Verification items for the finished model (mm, model axes). A direction names the side the tool comes from. Coordinates: 2 decimals unless noted, no trailing zeros. Order: outer loops, then holes, each group sorted by start corner. A loop starts at its lowest first (then second) coordinate and runs counter-clockwise, first axis right, second up. Notation, with made-up numbers: M 24,78 L 56,78 A22 ccw 56,86 Z; hole C 5.5,-30 d8. An arc over 180 degrees is marked long. Return JSON: item names as keys, results as strings. Group by question number.
1. Material ranges on line 1 along Y through (x, z) = (14.75, 5.75); line 2 along X through (y, z) = (5, 5); line 3 along Y through (x, z) = (-2, 6.5), recorded low to high.
2. Mould release check, pull along X, two halves, no side actions. Record for faces 5 (the cylindrical face through (-2, 10.5, 5)), 6 (the flat face through (8, 9, 0)), 7 (the flat face through (10, 16, 4)): +X half, -X half, draft (parallel to the pull), parting line (faces both ways), or undercut.
3. Section check C-C, the plane z = 1.75. Record the cut outline in (x, y), plus the area to 3 significant figures.
4. Section check B-B, the plane y = 12. Record the cut outline in (x, z), plus the area to 3 significant figures.
5. Gauge pin test, flat ends, axial feed: pin 1 (4 mm diameter, centred on y = 3.5, z = 2.5, fed in from +X); pin 2 (2.5 mm diameter, centred on x = -1.7, z = 4.15, fed in from -Y); pin 3 (4.5 mm diameter, centred on x = -1.5, z = 3.5, fed in from +Y). Record the tip position at first contact, or that the pin passes through.
6. Section check D-D, the plane x = 4. Record the cut outline in (y, z), plus the area to 3 significant figures.
7. Section check A-A, the plane x = 11.75. Record the cut outline in (y, z).
8. Set-up check for faces 1 (the flat face through (16.1, 5, 4)), 2 (the flat face through (0, 14, 4)), 3 (the flat face through (13, 14.6, 4)), 4 (the flat face through (0, 5, 4)): record each of +Z, -Z, +X, -X, +Y, -Y from which the full face is reachable in a straight line by a thin tool's end or side.
```python
from build123d import *

# Parameters (mm, degrees)
EXTRUDE_1_DEPTH     = 8.3
SKETCH_9_R          = 1.8
EXTRUDE_6_DEPTH     = 3
CHAMFER_1_SIZE      = 0.3
EXTRUDE_7_DEPTH     = 0.5
SKETCH_11_R         = 0.9
CUT_EXTRUDE_1_DEPTH = 10


with BuildPart() as part:
    # 草图1 → 凸台-拉伸1 (new body)
    with BuildSketch(Plane.XY):
        Polygon((16.1, 10.2), (17.8, 10.2), (17.8, 10.7), (16.1, 10.7), (16.1, 14.6), (10, 14.6), (10, 17.2), (0, 17.2), (0, 10.7), (-1.7, 10.7), (-1.7, 10.2), (0, 10.2), (0, 0), (16.1, 0), align=None)
    extrude(amount=EXTRUDE_1_DEPTH)

    # 草图9 → 凸台-拉伸6 (add)
    with BuildSketch(Plane(origin=(0, 17.2, 0), x_dir=(1, 0, 0), z_dir=(0, 1, 0))):
        with Locations(Location((4, -4, 0), (0, 0, 270))):
            Circle(SKETCH_9_R)
    extrude(amount=EXTRUDE_6_DEPTH)

    # 倒角1
    chamfer_1_edges = [part.edges().sort_by_distance(p)[0] for p in [
        (8.05, 0, 0),
        (0, 5.1, 0),
        (0, 13.95, 0),
        (5, 17.2, 0),
        (10, 15.9, 0),
        (13.05, 14.6, 0),
        (16.1, 12.65, 0),
        (16.1, 5.1, 0),
        (16.1, 12.65, 8.3),
        (16.1, 0, 4.15),
        (0, 0, 4.15),
        (0, 17.2, 4.15),
        (10, 17.2, 4.15),
        (10, 14.6, 4.15),
        (16.1, 14.6, 4.15),
        (13.05, 14.6, 8.3),
        (10, 15.9, 8.3),
        (5, 17.2, 8.3),
        (0, 13.95, 8.3),
        (16.1, 5.1, 8.3),
        (0, 5.1, 8.3),
        (8.05, 0, 8.3),
    ]]
    chamfer(chamfer_1_edges, length=CHAMFER_1_SIZE)

    # 草图10 → 凸台-拉伸7 (add)
    with BuildSketch(Plane(origin=(0, 10.7, 0), x_dir=(1, 0, 0), z_dir=(0, 1, 0))):
        with BuildLine():
            Line((-1.7, -8.3), (-1.7, 0))
            ThreePointArc((-1.7, 0), (-3.6, -4.15), (-1.7, -8.3))
        make_face()
        with BuildLine():
            ThreePointArc((19.7, -4.15), (19.202419193, -1.867868321), (17.8, 0))
            Line((17.8, 0), (17.8, -8.3))
            ThreePointArc((17.8, -8.3), (19.202419193, -6.432131679), (19.7, -4.15))
        make_face()
    extrude(amount=-EXTRUDE_7_DEPTH)

    # 草图11 → 切除-拉伸1 (cut)
    with BuildSketch(Plane(origin=(0, 10.7, 0), x_dir=(1, 0, 0), z_dir=(0, 1, 0))):
        with Locations(Location((-1.7, -4.15, 0), (0, 0, 270))):
            Circle(SKETCH_11_R)
        with Locations(Location((17.8, -4.15, 0), (0, 0, 270))):
            Circle(SKETCH_11_R)
    extrude(amount=-CUT_EXTRUDE_1_DEPTH, mode=Mode.SUBTRACT)


solid = part.part
```
Answers follow:
{
 "1": {"line 1": "0 to 14.6", "line 2": "0 to 16.1", "line 3": "10.2 to 10.7"},
 "2": {"face 5": "undercut", "face 6": "draft", "face 7": "+X half"},
 "3": {"outline": "M -3.05,10.2 L 0,10.2 L 0,0.3 L 0.3,0 L 15.8,0 L 16.1,0.3 L 16.1,10.2 L 19.15,10.2 L 19.15,10.7 L 16.1,10.7 L 16.1,14.3 L 15.8,14.6 L 10.3,14.6 L 10,14.9 L 10,16.9 L 9.7,17.2 L 0.3,17.2 L 0,16.9 L 0,10.7 L -3.05,10.7 Z", "area": "264 mm^2"},
 "4": {"outline": "M 0,0.3 L 0.3,0 L 15.8,0 L 16.1,0.3 L 16.1,8 L 15.8,8.3 L 0.3,8.3 L 0,8 Z", "area": "133 mm^2"},
 "5": {"pin 1": "x = 16.1", "pin 2": "y = 10.2", "pin 3": "y = 17.2"},
 "6": {"outline": "M 0,0.3 L 0.3,0 L 16.9,0 L 17.2,0.3 L 17.2,2.2 L 20.2,2.2 L 20.2,5.8 L 17.2,5.8 L 17.2,8 L 16.9,8.3 L 0.3,8.3 L 0,8 Z", "area": "153 mm^2"},
 "7": {"outline": "M 0,0.3 L 0.3,0 L 14.3,0 L 14.6,0.3 L 14.6,8 L 14.3,8.3 L 0.3,8.3 L 0,8 Z"},
 "8": {"face 1": "+Z, -Z, +X, -Y", "face 2": "+Z, -Z, -X, +Y", "face 3": "+Z, -Z, +X, +Y", "face 4": "+Z, -Z, -X, -Y"}
}
